The drawing under review shows one solid part. Ordinate dimensions are in mm from its lowest x, y, z. A direction names the side the tool comes from. Coordinates: 2 decimals unless noted, no trailing zeros. Order: outer loops, then holes, each group sorted by start corner. A loop starts at its lowest first (then second) coordinate and runs counter-clockwise, first axis right, second up. Notation, with made-up numbers: (69, 76) -> (77, 76) arc R19 cw to (77, 103) -> close; hole circle Ø10 at (-26.5, 63.5). An arc over 180 degrees is marked (long way). Write item = value, one per line.
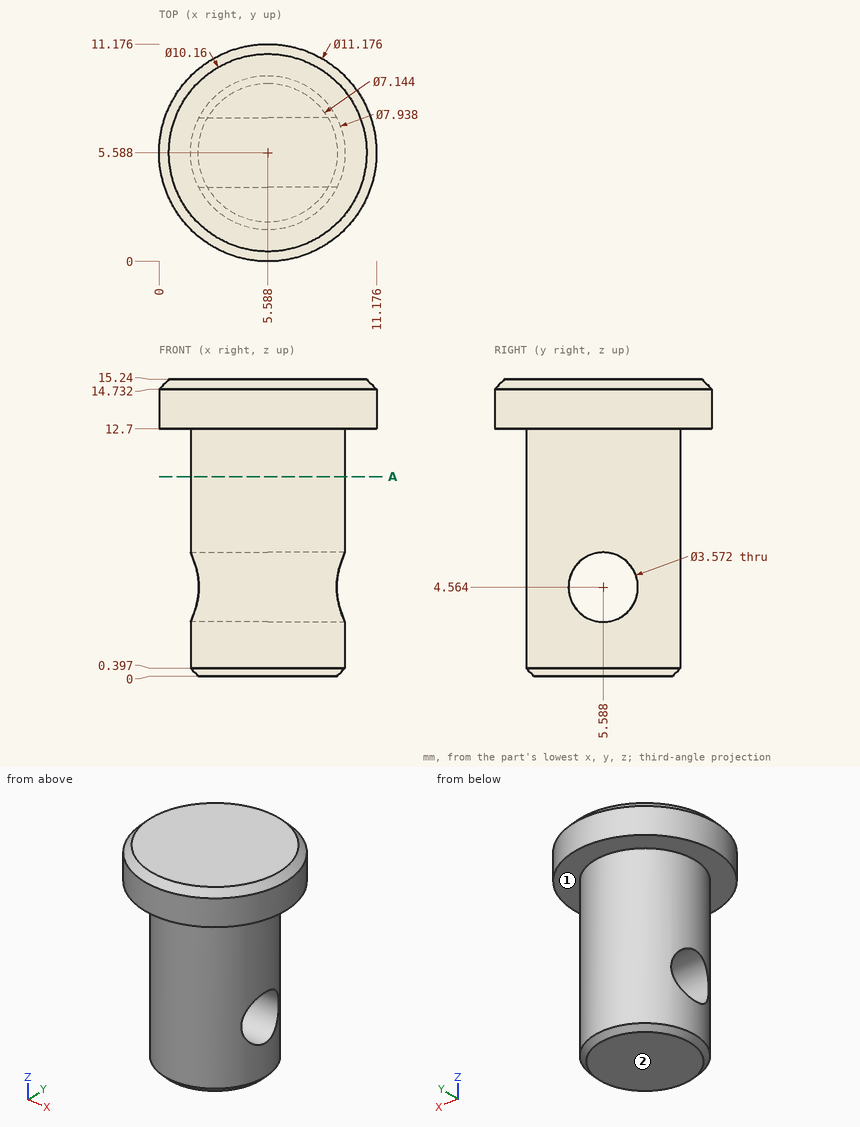
(1) For L1, parallel to Z at x = 10.25, y = 5.5; L2, parallel to Z at x = 7, y = 5.75 (1 decimal); L3, parallel to Z at x = 4.75, y = 5, list the stretches that pass through material, from the lowest coordinate up.
Report:
L1 = 12.7 to 15.24
L2 = 0 to 2.8, 6.3 to 15.2
L3 = 0 to 2.88, 6.25 to 15.24
(2) Insertion check: pin 1 (2 mm diameter, centred on y = 5.59, z = 4.56, fed in from -X). The pin has a flat end and moves straight along its axis. Give the tip position at first contact, or say it passes through.
Report:
pin_1 = through
(3) We need section A-A (z = 10.25). Write out the cut boundary in (x, y).
Report:
outline = circle Ø7.94 at (5.59, 5.59)
(4) For the marked faces 1 and 2, list the 3-axis set-ups (+Z, -Z, +X, -X, +Y, -Y) from which the entire face can be reached by the end or side of a thin tool; tool diameter is ignored.
Report:
face_1 = -Z
face_2 = -Z, +X, -X, +Y, -Y
